Part model, mm, in its own coordinate system. A direction names the side the tool comes from. Give positions to 0.01 mm unless a question says otherwise; leave off trailing zeros. Write each loop counter-clockwise with the first axis right and the second up, starting at its lowest first coordinate (ties: lowest second). Pieces come first, ordered by that corner, then holes. Notation, with made-up numbers: M 69,-4.75 L 94,-4.75 A17 ccw 94,3.25 Z; hole C -34,7 d1. An arc over 180 degrees is marked long. Use CSV: the item, a comma, the result in double quotes. Start each with the question number.
Item 1: Which spindle directions (+Z, -Z, +X, -X, +Y, -Y) get a long thin tool onto all of the face, cutting with end or side? Do faces 1 (the cylindrical face through (4.9, 3.4, -7.7)), 2 (the cylindrical face through (13.993, -8.246, -23.186)), 3 (the cylindrical face through (100.397, -5.246, -15.322)). Say none if no direction does.
Item 2: Cut at A-A (x = 167.5). List the corners of the cut face in (y, z), then the cut area to 3 significant figures.
Item 3: Cut at D-D (x = 139.5). List the corners of the cut face in (y, z).
Item 4: Pin check, flat tips, straight feed: pin 1 (2 mm diameter, centred on y = 2.5, z = -13, fed in from +X); pin 2 (7 mm diameter, centred on x = 97, z = -12, fed in from +Y); pin 3 (1.6 mm diameter, centred on x = 161, y = 1, fed in from +Z). Stop position of each tip, or through.
Item 5: Drill centre lines: line 1 (Z direction, x = 6.5, y = 3.45); line 2 (Z direction, x = 6.5, y = 1.5); line 3 (Z direction, x = 167.5, y = 2.15). Where is each one in solid material? Low to high. Write a range as [from, to].
Item 6: Mould opens along Y. For faces 4 (the flat face through (16, 9, -26)), 5 (the flat face through (95, -5, -18)), 6 (the cylindrical face through (165.5, 3.4, -35.1)), 7 (the flat face through (165, 2.8, -35)) say: released by +Y, released by -Y, zero draft, split by the parting line, or undercut.
Item 7: Cut at B-B (z = -6.5). List the corners of the cut face in (x, y), then the cut area to 3 significant figures.
Autodesk Inventor part; units mm, degrees
ref_plane "Płaszczyzna konstrukcyjna1" through (12.19341, -5.5, -26.646) normal (0, -1, 0) x (1, 0, 0)
ref_plane "Płaszczyzna konstrukcyjna2" through (12.19341, -9, -26.646) normal (0, -1, 0) x (1, 0, 0)
ref_plane "Płaszczyzna konstrukcyjna3" through (96.2, -5.5, -14) normal (0, -1, 0) x (1, 0, 0)
sketch "Szkic1" plane through (0, 0, 0) normal (0, 1, 0) x (-1, 0, 0)
  line L0 (0, 0) -> (-174, 0)
  line L1 (-174, 0) -> (-174, -41.646)
  line L2 (-174, -41.646) -> (0, -41.646)
  line L3 (0, -41.646) -> (0, 0)
  dimension "d0" = 174
  dimension "d1" = 41.646
extrude "Wyciągnięcie proste1" add sketch "Szkic1" along normal blind 2
sketch "Szkic2" plane through (0, 2, 0) normal (0, 1, 0) x (1, 0, 0)
  line L0 (174, 41.646) -> (0, 41.646)
  line L1 (174, 0) -> (174, 41.646)
  line L2 (174, 41.646) -> (0, 41.646)
  line L3 (0, 41.646) -> (0, 0)
  line L4 (0, 0) -> (174, 0)
  line L5 (171, 23) -> (171, 38.646)
  line L6 (2.5, 38.646) -> (2.5, 3)
  line L7 (2.5, 3) -> (153.5, 3)
  line L8 (2.5, 41.646) -> (2.5, 38.646)
  line L9 (127, 41.646) -> (47, 41.646)
  line L10 (153.5, 19) -> (171, 19)
  line L11 (171, 19) -> (171, 23)
  line L12 (153.5, 19) -> (153.5, 3)
  line L13 (127, 38.646) -> (127, 41.646)
  line L14 (2.5, 38.646) -> (47, 38.646)
  line L15 (127, 38.646) -> (171, 38.646)
  line L16 (47, 38.646) -> (47, 41.646)
  dimension "d4" = 3
  dimension "d122" = 17.5
  dimension "d123" = 16
  dimension "d150" = 3
  dimension "d151" = 44.5
extrude "Wyciągnięcie proste2" add sketch "Szkic2" along normal blind 2 contours L13 L15 L5 L11 L10 L12 L7 L6 L14 L16 L0
sketch "Szkic21" plane through (0, 0, 0) normal (0, -1, 0) x (1, 0, 0)
  line L0 (0, -41.646) -> (0, 0)
  line L1 (0, -41.646) -> (0, 0)
  line L2 (0, -26.646) -> (12, -26.646)
  line L3 (174, -41.646) -> (0, -41.646)
  line L4 (12, -41.646) -> (12, -26.646)
  circle A0 centre (12, -26.646) radius 3.9
  dimension "d90" = 12
  dimension "d91" = 15
  dimension "d92" = 7.8
extrude "Wyciągnięcie proste20" add sketch "Szkic21" along normal blind 5 contours A0 L4 L2 | L2 L4 A0
sketch "Szkic22" plane through (12, -5, -26.646) normal (0, -1, 0) x (1, 0, 0)
  circle A0 centre (0, 0) radius 3.9
  circle A1 centre (0.19341, 0) radius 4.4
  point P0 (-12, 26.646)
  dimension "d95" = 8.8
extrude "Wyciągnięcie proste21" add sketch "Szkic22" along normal blind 0.5 contours A0 | A1
ref_plane "Płaszczyzna konstrukcyjna1" through (12.19341, -5.5, -26.646) normal (0, -1, 0) x (1, 0, 0)
sketch "Szkic23" plane through (12.19341, -5.5, -26.646) normal (0, -1, 0) x (1, 0, 0)
  circle A0 centre (0, 0) radius 4.4
  circle A1 centre (0, 0) radius 4.4
  point P0 (-12.19341, 26.646)
extrude "Wyciągnięcie proste22" add sketch "Szkic23" along normal blind 2.5 draft -11.31
sketch "Szkic24" plane through (12.19341, -8, -26.646) normal (0, -1, 0) x (1, 0, 0)
  circle A0 centre (0, 0) radius 3.899997
  circle A1 centre (0, 0) radius 3.899997
  point P0 (-12.19341, 26.646)
extrude "Wyciągnięcie proste23" add sketch "Szkic24" along normal blind 0.5
sketch "Szkic25" plane through (12.19341, -8.5, -26.646) normal (0, -1, 0) x (1, 0, 0)
  circle A0 centre (0, 0) radius 4.4
  circle A1 centre (0, 0) radius 4.4
  point P0 (-12.19341, 26.646)
extrude "Wyciągnięcie proste24" add sketch "Szkic25" along normal blind 0.5
ref_plane "Płaszczyzna konstrukcyjna2" through (12.19341, -9, -26.646) normal (0, -1, 0) x (1, 0, 0)
sketch "Szkic26" plane through (12.19341, -9, -26.646) normal (0, -1, 0) x (1, 0, 0)
  circle A0 centre (0, 0) radius 4.4
  circle A1 centre (0, 0) radius 4.4
  point P0 (-12.19341, 26.646)
extrude "Wyciągnięcie proste25" add sketch "Szkic26" along normal blind 2.5 draft -11.31
sketch "Szkic27" plane through (12.19341, -11.5, -26.646) normal (0, -1, 0) x (1, 0, 0)
  circle A0 centre (0, 0) radius 3.899997
  circle A1 centre (0, 0) radius 3.25
  point P0 (-12.19341, 26.646)
  dimension "d108" = 6.5
extrude "Wyciągnięcie proste26" cut sketch "Szkic27" against normal blind 32 contours A1
mirror "Odbij1" about plane through (87, 2, -20.823) normal (0, 1, 0) of "Wyciągnięcie proste20", "Wyciągnięcie proste21", "Wyciągnięcie proste22", "Wyciągnięcie proste24", "Wyciągnięcie proste25", "Wyciągnięcie proste26", "Wyciągnięcie proste23"
sketch "Szkic28" plane through (0, 0, 0) normal (0, -1, 0) x (1, 0, 0)
  line L0 (174, 0) -> (174, -41.646)
  line L1 (174, 0) -> (156, 0)
  line L2 (156, 0) -> (156, -16)
  line L3 (156, -16) -> (174, -16)
  line L4 (174, -16) -> (174, 0)
  point P0 (0, 0)
  dimension "d111" = 18
  dimension "d112" = 16
extrude "Wyciągnięcie proste27" cut sketch "Szkic28" against normal blind 4
sketch "Szkic29" plane through (0, 0, 0) normal (0, -1, 0) x (1, 0, 0)
  line L0 (0, 0) -> (156, 0)
  line L1 (0, 0) -> (96.2, 0)
  line L2 (96.2, 0) -> (96.2, -14)
  circle A0 centre (96.2, -14) radius 3.9
  dimension "d124" = 96.2
  dimension "d125" = 14
  dimension "d126" = 7.8
extrude "Wyciągnięcie proste28" add sketch "Szkic29" along normal blind 5
sketch "Szkic30" plane through (96.2, -5, -14) normal (0, -1, 0) x (1, 0, 0)
  circle A0 centre (0, 0) radius 3.9
  circle A1 centre (0, 0) radius 4.4
  point P0 (-96.2, 14)
  dimension "d129" = 8.8
extrude "Wyciągnięcie proste29" add sketch "Szkic30" along normal blind 0.5 contours A0 | A1
ref_plane "Płaszczyzna konstrukcyjna3" through (96.2, -5.5, -14) normal (0, -1, 0) x (1, 0, 0)
sketch "Szkic31" plane through (96.2, -5.5, -14) normal (0, -1, 0) x (1, 0, 0)
  circle A0 centre (0, 0) radius 4.4
  circle A1 centre (0, 0) radius 4.4
  point P0 (-96.2, 14)
extrude "Wyciągnięcie proste30" add sketch "Szkic31" along normal blind 2.5 draft -11.31
sketch "Szkic32" plane through (96.2, -8, -14) normal (0, -1, 0) x (1, 0, 0)
  circle A0 centre (0, 0) radius 3.899997
  point P0 (-96.2, 14)
extrude "Wyciągnięcie proste31" add sketch "Szkic32" along normal blind 0.5
sketch "Szkic33" plane through (96.2, -8.5, -14) normal (0, -1, 0) x (1, 0, 0)
  circle A0 centre (0, 0) radius 4.4
  circle A1 centre (0, 0) radius 4.4
  point P0 (-96.2, 14)
extrude "Wyciągnięcie proste32" add sketch "Szkic33" along normal blind 0.5
ref_plane "Płaszczyzna konstrukcyjna4" through (96.2, -9, -14) normal (0, -1, 0) x (1, 0, 0)
sketch "Szkic34" plane through (96.2, -9, -14) normal (0, -1, 0) x (1, 0, 0)
  circle A0 centre (0, 0) radius 3.9
  circle A1 centre (0, 0) radius 4.4
  point P0 (-96.2, 14)
sketch "Szkic34 outline for Wyciągnięcie proste33" plane through (96.2, -9, -14) normal (0, -1, 0) x (1, 0, 0)
  circle A0 centre (0, 0) radius 4.4
extrude "Wyciągnięcie proste33" add sketch "Szkic34 outline for Wyciągnięcie proste33" along normal blind 2.5 draft -11.31
sketch "Szkic35" plane through (96.2, -11.5, -14) normal (0, -1, 0) x (1, 0, 0)
  circle A0 centre (0, 0) radius 3.25
  point P0 (-96.2, 14)
  dimension "d142" = 6.5
extrude "Wyciągnięcie proste34" cut sketch "Szkic35" against normal blind 16
sketch "Szkic37" plane through (0, 0, 0) normal (0, -1, 0) x (1, 0, 0)
  line L0 (0, 0) -> (156, 0)
  line L1 (2.5, -3) -> (153.5, -3)
  line L2 (0, -6.5) -> (6.5, -6.5)
  line L3 (6.5, 0) -> (6.5, -6.5)
  line L4 (0, -41.646) -> (0, 0)
  circle A0 centre (6.5, -6.5) radius 3
  line L5 (0, -20.823) -> (4.213625, -20.823)
  circle A1 centre (6.5, -35.146) radius 3
  line L6 (174, -41.646) -> (0, -41.646)
  line L7 (87, -41.646) -> (87, -34.846)
  circle A2 centre (167.5, -35.146) radius 3
  line L8 (2.5, -3) -> (78, -3)
  line L9 (78, -3) -> (78, -5.430935)
  circle A3 centre (149.5, -6.5) radius 3
  dimension "d156" = 6.5
  dimension "d160" = 6.5
  dimension "d161" = 6
extrude "Wyciągnięcie proste37" cut sketch "Szkic37" against normal blind 2.8 contours A0 L3 L2 | L2 L3 A0 | A1 | A2 | A3
sketch "Szkic38" plane through (6.5, 2.8, -6.5) normal (0, -1, 0) x (1, 0, 0)
  circle A0 centre (0, 0) radius 2
  line L0 (-6.5, -35.146) -> (-6.5, 6.5)
  line L1 (-6.5, -14.323) -> (-2.3, -14.323)
  circle A1 centre (0, -28.646) radius 2
  line L2 (167.5, -35.146) -> (-6.5, -35.146)
  line L3 (80.5, -35.146) -> (80.5, -30.046)
  circle A2 centre (161, -28.646) radius 2
  line L4 (-4, 3.5) -> (147, 3.5)
  line L5 (-4, 3.5) -> (71.5, 3.5)
  line L6 (71.5, 3.5) -> (71.5, -1.9)
  circle A3 centre (143, 0) radius 2
  dimension "d164" = 4
extrude "Wyciągnięcie proste38" cut sketch "Szkic38" against normal blind 3
sketch "Szkic39" plane through (0, 0, 0) normal (0, -1, 0) x (1, 0, 0)
  circle A0 centre (149.5, -6.5) radius 3
  line L0 (146.5, -6.5) -> (131.5, -6.5)
  circle A1 centre (131.5, -6.5) radius 2.5
  point P0 (0, 0)
  dimension "d167" = 15
  dimension "d168" = 5
extrude "Wyciągnięcie proste39" cut sketch "Szkic39" against normal blind 10 contours A1
properties part number "Klapa_Drukowanie 3D"
Worked answers:
1,face 1,"+Y, -Y"
1,face 2,"none"
1,face 3,"-Y"
2,outline,"M 0,-41.65 L 2,-41.65 L 2,-38.65 L 4,-38.65 L 4,-37.15 L 2.8,-37.15 L 2.8,-38.15 L 0,-38.15 Z; M 0,-32.15 L 2.8,-32.15 L 2.8,-33.15 L 4,-33.15 L 4,-19 L 2,-19 L 2,-16 L 0,-16 Z"
2,area,"69.0 mm^2"
3,outline,"M 0,-41.65 L 2,-41.65 L 2,-38.65 L 4,-38.65 L 4,-3 L 2,-3 L 2,0 L 0,0 Z"
4,pin 1,"stops at x = 156"
4,pin 2,"stops at y = 4"
4,pin 3,"stops at z = -16"
5,line 1,"z = [-38.65, -37.15], [-33.15, -8.5], [-4.5, -3]"
5,line 2,"z = [-41.65, -38.15], [-32.15, -9.5], [-3.5, 0]"
5,line 3,"z = [-38.65, -38.15], [-32.15, -19]"
6,face 4,"undercut"
6,face 5,"undercut"
6,face 6,"zero draft"
6,face 7,"released by -Y"
7,outline,"M 0,0 L 3.5,0 L 3.5,2.8 L 4.5,2.8 L 4.5,4 L 2.5,4 L 2.5,2 L 0,2 Z; M 8.5,2.8 L 9.5,2.8 L 9.5,0 L 129,0 L 129,4 L 8.5,4 Z; M 134,0 L 146.5,0 L 146.5,2.8 L 147.5,2.8 L 147.5,4 L 134,4 Z; M 151.5,2.8 L 152.5,2.8 L 152.5,0 L 156,0 L 156,2 L 153.5,2 L 153.5,4 L 151.5,4 Z"
7,area,"551 mm^2"
